```python
from build123d import *

# Parameters (mm, degrees)
SKETCH1_R                   = 95.25
BOSS_EXTRUDE1_DEPTH         = 4.7625
M2X0_4_TAPPED_HOLE1_D       = 1.6
M2X0_4_TAPPED_HOLE1_DEPTH   = 5.334
M2X0_4_TAPPED_HOLE2_D       = 1.6
M2X0_4_TAPPED_HOLE2_DEPTH   = 5.334
F_1_2_13_TAPPED_HOLE1_D     = 10.71626
F_1_2_13_TAPPED_HOLE1_DEPTH = 31.242


with BuildPart() as part:
    # Sketch1 → Boss-Extrude1 (new body)
    with BuildSketch(Plane.XY):
        Circle(SKETCH1_R)
    extrude(amount=BOSS_EXTRUDE1_DEPTH)

    # M2x0.4 Tapped Hole1
    with Locations(Plane.XY.offset(4.7625)):
        with Locations((-83.278324724, 33.02), (-68.038324724, 33.02), (-72.688137364, 50.8), (-57.448137364, 50.8), (-89.542383388, 10.16), (-74.302383388, 10.16), (-57.448137364, -50.8), (-72.688137364, -50.8), (-68.038324724, -33.02), (-83.278324724, -33.02), (-74.302383388, -10.16), (-89.542383388, -10.16), (57.448137364, -50.8), (72.688137364, -50.8), (68.038324724, -33.02), (83.278324724, -33.02), (89.542383388, -10.16), (74.302383388, -10.16), (89.542383388, 10.16), (74.302383388, 10.16), (83.278324724, 33.02), (68.038324724, 33.02), (57.448137364, 50.8), (72.688137364, 50.8)):
            Hole(M2X0_4_TAPPED_HOLE1_D / 2, depth=M2X0_4_TAPPED_HOLE1_DEPTH)

    # M2x0.4 Tapped Hole2
    with Locations(Plane.XY.offset(4.7625)):
        with Locations((-41.275, -63.5), (-9.525, -63.5), (9.525, -63.5), (41.275, -63.5), (-15.875, 69.85), (15.875, 69.85)):
            Hole(M2X0_4_TAPPED_HOLE2_D / 2, depth=M2X0_4_TAPPED_HOLE2_DEPTH)

    # 1/2-13 Tapped Hole1
    with Locations(Plane.XY.offset(4.7625)):
        with Locations((0, 69.85), (-25.4, -63.5), (25.4, -63.5)):
            Hole(F_1_2_13_TAPPED_HOLE1_D / 2, depth=F_1_2_13_TAPPED_HOLE1_DEPTH)


solid = part.part
```
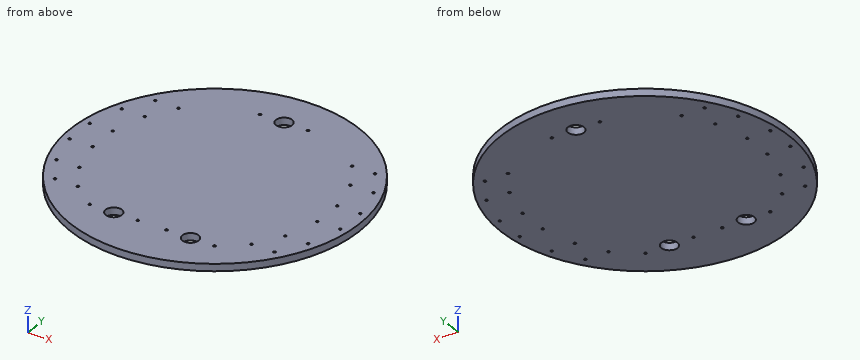
The listing builds one solid part. Answer for the finished solid, in the listing's coordinates (mm). Give positions to 0.01 mm unless a question says otherwise; leave off trailing zeros. Loops run counter-clockwise (first coordinate to the right, second up) from the corner with the lowest first, then second, coordinate; pieces in that order, holes last. Notation, with made-up numbers: M 34,16.25 L 79,16.25 A22 ccw 79,22.25 Z; hole C 75.25,83 d4. An arc over 180 degrees is marked long. One line per item, written item: value.
1. Section D-D on y = 42.5 is taken. Determine the outline of the cut face in (x, z), plus the area to 3 significant figures.
Found:
outline: M -85.24,0 L 85.24,0 L 85.24,4.76 L -85.24,4.76 Z
area: 812 mm^2
2. Section C-C on y = -81 is taken. Determine the outline of the cut face in (x, z).
Found:
outline: M -50.12,0 L 50.12,0 L 50.12,4.76 L -50.12,4.76 Z
3. Section A-A on x = 0 is taken. Determine the outline of the cut face in (y, z).
Found:
outline: M -95.25,0 L 64.49,0 L 64.49,4.76 L -95.25,4.76 Z; M 75.21,0 L 95.25,0 L 95.25,4.76 L 75.21,4.76 Z
4. Find the intervals of material crossed by probe 1 along X at (y, z) = (-50.8, 3.4); probe 2 along Y at (x, z) = (75, 2.3); probe 3 along X at (y, z) = (-33, 0.8), in increasing order.
Found:
probe 1: -80.57 to -73.49, -71.89 to -58.25, -56.65 to 56.65, 58.25 to 71.89, 73.49 to 80.57
probe 2: -58.72 to -10.55, -9.77 to 9.77, 10.55 to 58.72
probe 3: -89.35 to -84.08, -82.48 to -68.84, -67.24 to 67.24, 68.84 to 82.48, 84.08 to 89.35
5. Section B-B on z = 1.1 is taken. State how many separate pieces and enclosed holes the cut face has, plus the area to 3 significant figures.
Found:
separate pieces: 1
enclosed holes: 33
area: 28,200 mm^2
